CAD build for the part. Positions are in the model's coordinates, mm. Face numbers are marked on the shaded views. Give positions to 0.01 mm unless a question says otherwise; leave off trailing zeros. Order: outer loops, then holes, each group sorted by start corner. A loop starts at its lowest first (then second) coordinate and runs counter-clockwise, first axis right, second up.
Autodesk Inventor part; units mm, degrees
ref_plane "Work Plane1" through (-3.92, -29.81, 0) normal (-1, 0, 0) x (0, 0, 1)
ref_plane "YZ Plane" through (0, 0, 0) normal (1, 0, 0) x (0, 1, 0)
ref_plane "XZ Plane" through (0, 0, 0) normal (0, 1, 0) x (-1, 0, 0)
sketch "Sketch1" plane through (0, 0, 0) normal (0, 0, 1) x (1, 0, 0)
  line L0 (-21.1, 29.81) -> (21.1, 29.81)
  line L1 (21.1, 29.81) -> (21.1, -29.81)
  line L2 (21.1, -29.81) -> (-21.1, -29.81)
  line L3 (-21.1, -29.81) -> (-21.1, 29.81)
  line L4 (0, 0) -> (0, 68.2086)
  line L5 (0, 0) -> (53.7664, 0)
  dimension "d0" = 59.62
  dimension "d1" = 42.2
extrude "Extrusion1" add sketch "Sketch1" along normal blind 30.3
ref_plane "Work Plane1" through (-3.92, -29.81, 0) normal (-1, 0, 0) x (0, 0, 1)
sketch "Sketch3" plane through (-3.92, -29.81, 0) normal (-1, 0, 0) x (0, 0, 1)
  line L0 (0, 59.62) -> (30.3, 59.62)
  line L1 (30.3, 59.62) -> (30.3, 0)
  line L2 (30.3, 44.35) -> (38.03, 44.35)
  line L3 (39.0073, 54.42) -> (18.3537, 54.42)
  arc A0 (30.3, 34.28) -> (30.3, 54.42) centre (27.6058, 44.35) ccw
  point P0 (0, 29.81)
  dimension "d8" = 7.73
  dimension "d9" = 15.27
  dimension "d10" = 5.2
  dimension "d11" = 20.14
revolve "Revolution1" add sketch "Sketch3" angle 360 about axis through (-3.92, 14.54, 30.3) along (0, 0, 1) picked at (31.0054, 37.9107) contours L2 A0 L1
sketch "Sketch6" plane through (0, 0, 30.3) normal (0, 0, 1) x (1, 0, 0)
  circle A0 centre (-3.92, 14.54) radius 10.07
  circle A1 centre (-3.92, 14.54) radius 10.07
  point P0 (0, 0)
extrude "Extrusion4" add sketch "Sketch6" along normal blind 5.43
sketch "Sketch7" plane through (21.1, -29.81, 0) normal (1, 0, 0) x (0, 0, -1)
  line L0 (-35.73, 34.28) -> (-35.73, 54.42)
  line L1 (-35.73, 54.42) -> (-46.1148, 54.42)
  line L2 (-46.1148, 54.42) -> (-46.1148, 34.28)
  line L3 (-46.1148, 34.28) -> (-35.73, 34.28)
  line L4 (-35.73, 34.28) -> (-35.73, 54.42)
  point P0 (0, 29.81)
extrude "Extrusion5" cut sketch "Sketch7" against normal blind 400
sketch "Sketch8" plane through (-3.92, -29.81, 0) normal (-1, 0, 0) x (0, 0, 1)
  line L0 (35.73, 54.42) -> (35.73, 34.28)
  line L1 (35.73, 44.35) -> (38.6, 44.35)
  line L2 (31.2686, 37.15) -> (43.7794, 37.15)
  line L3 (30.3, 34.28) -> (35.73, 34.28)
  line L4 (31.2686, 51.55) -> (47.0475, 51.55)
  line L5 (30.3, 54.42) -> (35.73, 54.42)
  arc A0 (35.73, 37.15) -> (35.73, 51.55) centre (28.1336, 44.35) ccw
  point P0 (0, 29.81)
  dimension "d27" = 2.87
  dimension "d28" = 2.87
  dimension "d29" = 2.87
revolve "Revolution2" add sketch "Sketch8" angle 360 about axis through (-3.92, 14.54, 35.73) along (0, 0, 1) picked at (36.137, 48.6296) contours A0 L1 L0
sketch "Sketch9" plane through (-3.92, -29.81, 0) normal (-1, 0, 0) x (0, 0, 1)
  line L0 (35.73, 54.42) -> (35.73, 34.28)
  line L1 (30.3, 54.42) -> (30.3, 34.28)
  line L2 (35.73, 51.55) -> (35.73, 37.15)
  line L3 (31.5731, 44.35) -> (78.5809, 125.77)
  line L4 (31.5731, 44.35) -> (78.5809, -37.07)
  line L5 (30.3, 44.35) -> (31.5731, 44.35) construction
  point P0 (0, 29.81)
  point P1 (38.6, 44.35)
  dimension "d31" = 120
sketch "Sketch10" plane through (0, 0, 30.3) normal (0, 0, 1) x (1, 0, 0)
  circle A0 centre (-3.92, 14.54) radius 10.07
  line L0 (21.1, 29.81) -> (21.1, -29.81)
  line L1 (-21.1, 29.81) -> (21.1, 29.81)
  line L2 (-21.1, -29.81) -> (-21.1, 29.81)
  line L3 (21.1, -29.81) -> (-21.1, -29.81)
  point P0 (0, 0)
properties part number "Camera" material "PVC-Piping"
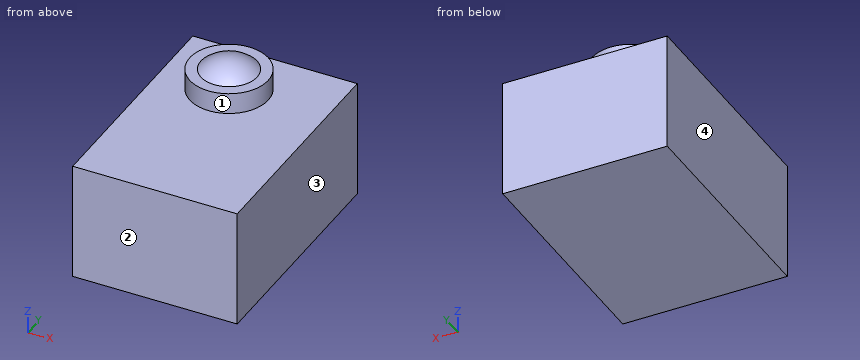
Item 1: Wall check: L1, parallel to Z at x = -3, y = -26; L2, parallel to Z at x = -10, y = 15.5; L3, parallel to Y at x = -2.5, z = 34. Give the ranges that are in metal, low to high.
Item 2: Slice it at C-C (z = 33). Give the cut face in (x, y), and give its area (3 significant figures).
Item 3: Drop flat-ended pins along their axis: pin 1 Ø8 at (x, y) = (-10, -2) entering from +Z; pin 2 Ø21 at (x, y) = (-5, 1) entering from +Z. Give the stop position or say it passes through.
Item 4: Slice it at A-A (y = 14.54). Give the cut face in (x, z), and give its area (3 significant figures).
Item 5: Slice it at D-D (y = -23). Give the cut face in (x, z), and give its area (3 significant figures).
Item 6: Two-plate mould, pull along X, no slides. Class the marked faces 1, 2, 3 and 4: released by +X, released by -X, zero draft, split by the parting line, or undercut.
Item 7: Slice it at B-B (x = -3.92). Give the cut face in (y, z).
A:
1. L1: z = 0 to 30.3
1. L2: z = 0 to 36.6
1. L3: y = 4.57 to 24.51
2. outline: circle Ø20.14 at (-3.92, 14.54)
2. area: 319 mm2
3. pin 1: stops at z = 30.3
3. pin 2: stops at z = 38.14
4. outline: (-21.1, 0) - (21.1, 0) - (21.1, 30.3) - (6.15, 30.3) - (6.15, 35.73) - (3.28, 35.73) arc R10.47 ccw to (-11.12, 35.73) - (-13.99, 35.73) - (-13.99, 30.3) - (-21.1, 30.3) - close
4. area: 1,420 mm2
5. outline: (-21.1, 0) - (21.1, 0) - (21.1, 30.3) - (-21.1, 30.3) - close
5. area: 1,280 mm2
6. face 1: split by the parting line
6. face 2: zero draft
6. face 3: released by +X
6. face 4: released by -X
7. outline: (-29.81, 0) - (29.81, 0) - (29.81, 30.3) - (24.61, 30.3) - (24.61, 35.73) - (21.74, 35.73) arc R10.47 ccw to (7.34, 35.73) - (4.47, 35.73) - (4.47, 30.3) - (-29.81, 30.3) - close
